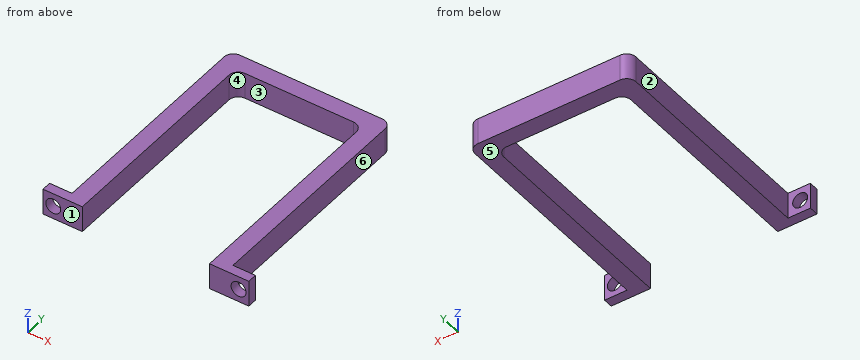
Autodesk Fusion 360 part; units mm, degrees
sketch "Sketch1" plane through (0, 0, 0) normal (0, 0, 1) x (1, 0, 0)
  line L0 (-27.5, 0) -> (27.5, 0)
  line L1 (-27.5, 0) -> (-27.5, 2.5)
  line L2 (-27.5, 2.5) -> (-21.5, 2.5)
  line L3 (0, 0) -> (0, 60)
  line L4 (27.5, 2.5) -> (21.5, 2.5)
  line L5 (0, 2.5) -> (-14, 2.5)
  line L6 (0, 2.5) -> (14, 2.5)
  line L7 (-14, 0) -> (-14, 2.5)
  line L8 (14, 2.5) -> (14, 0)
  line L9 (-14, 2.5) -> (-14, 62.5)
  line L10 (14, 2.5) -> (14, 62.5)
  line L11 (-21.5, 2.5) -> (-21.5, 62.5)
  line L12 (21.5, 2.5) -> (21.5, 62.5)
  line L13 (-21.5, 62.5) -> (21.5, 62.5)
  line L14 (0, 60) -> (-14, 60)
  line L15 (0, 60) -> (14, 60)
  line L16 (27.5, 2.5) -> (27.5, 0)
  dimension "d8" = 55
  dimension "d9" = 6
  dimension "d10" = 60
  dimension "d11" = 60
  dimension "d12" = 60
extrude "Extrude1" add sketch "Sketch1" along normal blind 7 contours L0 L1 L2 L7 L9 L11 L13 | L0 L4 L8 L10 L12 L13 L16 | L9 L10 L13 L14 L15
extrude "Extrude2" add 1 faces at (-4.6667, 60, 2.3333) along direction (0, -1, 0) blind 2
sketch "Sketch2" plane through (0, 62.5, 0) normal (0, 1, 0) x (-1, 0, 0)
  line L0 (-21.5, 0) -> (21.5, 0)
  line L1 (21.5, 0) -> (21.5, 7)
  line L2 (21.5, 7) -> (-21.5, 7)
  line L3 (-21.5, 7) -> (-21.5, 0)
  line L4 (0, 3.5) -> (24.765, 3.5)
  line L5 (0, 0) -> (0, 7)
  line L6 (0, 3.5) -> (-24.765, 3.5)
  circle A0 centre (24.765, 3.5) radius 2
  circle A1 centre (-24.765, 3.5) radius 2
  dimension "d17" = 24.765
  dimension "d18" = 4
  dimension "d19" = 4
extrude "Extrude3" cut sketch "Sketch2" against normal blind 66 contours A1 | A0
extrude "Extrude4" cut 1 faces at (-14, 19.3333, 4.6667) along direction (-1, 0, 0) blind 3
extrude "Extrude5" cut 1 faces at (14, 38.6667, 2.3333) along direction (1, 0, 0) blind 3
fillet "Fillet1" radius 2.5 1 edges at (-17, 58, 3.5)
fillet "Fillet2" radius 2.5 1 edges at (17, 58, 3.5)
fillet "Fillet3" radius 2.5 1 edges at (-21.5, 62.5, 3.5)
fillet "Fillet4" radius 2.5 1 edges at (21.5, 62.5, 3.5)
Source: CAD feature listing. Evaluate the final solid. Frame: model axes, mm. Face numbers are marked on the shaded views. A direction names the side the tool comes from. Coordinates: 2 decimals unless noted, no trailing zeros. Write each loop counter-clockwise with the first axis right and the second up, starting at its lowest first coordinate (ties: lowest second). Pieces come first, ordered by that corner, then holes. Notation, with made-up numbers: M -38.75,-25.5 L -33.75,-25.5 A18 ccw -33.75,-10.5 Z; hole C 61.5,-37.5 d9. An arc over 180 degrees is marked long. Use a Markdown table: item, result.
1) Section D-D, the plane x = 0. Output: boundary loops of the cut face in (y, z).
Conclusion:
| item | result |
|---|---|
| outline | M 58,0 L 62.5,0 L 62.5,7 L 58,7 Z |
2) Section C-C, the plane x = 23.5. Output: boundary loops of the cut face in (y, z), then the cut area to 3 significant figures.
Conclusion:
| item | result |
|---|---|
| outline | M 0,0 L 2.5,0 L 2.5,1.95 L 0,1.95 Z; M 0,5.05 L 2.5,5.05 L 2.5,7 L 0,7 Z |
| area | 9.75 mm^2 |
3) Ray query, L1, parallel to X at y = 47, z = 5.25; L2, parallel to Y at x = 1, z = 2.75; L3, parallel to Y at x = -23, z = 6.5. Return the intervals inside material, ascending.
Conclusion:
| item | result |
|---|---|
| L1 | x = -21.5 to -17, 17 to 21.5 |
| L2 | y = 58 to 62.5 |
| L3 | y = 0 to 2.5 |
4) Mould query, pull axis X, two halves, no side actions, for the marked faces 1, 2 and 3. Classes: pulls with the +X half, pulls with the -X half, needs draft (parallel to the pull), parting line crosses it, or undercut.
Conclusion:
| item | result |
|---|---|
| face 1 | needs draft |
| face 2 | pulls with the -X half |
| face 3 | undercut |
5) First-contact query: pin 1 Ø1 at (x, z) = (-11.5, 3) entering from -Y; pin 2 Ø3 at (x, z) = (-24.765, 3.5) entering from -Y; pin 3 Ø3.5 at (y, z) = (14, 2) entering from +X; pin 4 Ø3.5 at (y, z) = (41, 4) entering from -X. Flat tips, straight axial feed; report the tip coordinate or a pass-through.
Conclusion:
| item | result |
|---|---|
| pin 1 | stops at y = 58 |
| pin 2 | passes through |
| pin 3 | stops at x = 21.5 |
| pin 4 | stops at x = -21.5 |
6) Section A-A, the plane y = 28.5. Output: boundary loops of the cut face in (x, z).
Conclusion:
| item | result |
|---|---|
| outline | M -21.5,0 L -17,0 L -17,7 L -21.5,7 Z; M 17,0 L 21.5,0 L 21.5,7 L 17,7 Z |
7) Section B-B, the plane z = 3.5. Output: boundary loops of the cut face in (x, y) (3 decimals), then the cut area to 4 significant figures.
Conclusion:
| item | result |
|---|---|
| outline | M -27.5,0 L -26.765,0 L -26.765,2.5 L -27.5,2.5 Z; M -22.765,0 L -17,0 L -17,55.5 A2.5 cw -14.5,58 L 14.5,58 A2.5 cw 17,55.5 L 17,0 L 22.765,0 L 22.765,2.5 L 21.5,2.5 L 21.5,60 A2.5 ccw 19,62.5 L -19,62.5 A2.5 ccw -21.5,60 L -21.5,2.5 L -22.765,2.5 Z; M 26.765,0 L 27.5,0 L 27.5,2.5 L 26.765,2.5 Z |
| area | 725.5 mm^2 |
8) Reachability of the marked faces 4, 5 and 6 from +Z, -Z, +X, -X, +Y, -Y: full face, straight path, thin tool, end or side. Return the list, or none.
Conclusion:
| item | result |
|---|---|
| face 4 | +Z, -Z, -Y |
| face 5 | -Z, +X, -X, +Y, -Y |
| face 6 | +Z, -Z, +X, +Y |
